from build123d import *

# Parameters (mm, degrees)
SKETCH_W             = 57
SKETCH_H             = 69
PAD_DEPTH            = 9
SKETCH001_W          = 13.25
SKETCH001_H          = 16.25
POCKET_DEPTH         = 8
SKETCH002_W          = 2
SKETCH002_H          = 51.95
SKETCH002_W_2        = 42.95
SKETCH002_H_2        = 2
POCKET015_DEPTH      = 6
BODY_PLACEMENT_ANGLE = 90


with BuildPart() as part:
    # Sketch → Pad (new body)
    with BuildSketch(Plane.XY):
        with Locations((28.5, 34.5)):
            Rectangle(SKETCH_W, SKETCH_H)
    extrude(amount=PAD_DEPTH)

    # Sketch001 (on Face6 of Pad) → Pocket (cut)
    with BuildSketch(Plane.XY.offset(9)):
        with Locations((7.425, 60.075)):
            Rectangle(SKETCH001_W, SKETCH001_H)
        with Locations((21.475, 60.075)):
            Rectangle(SKETCH001_W, SKETCH001_H)
        with Locations((35.525, 60.075)):
            Rectangle(SKETCH001_W, SKETCH001_H)
        with Locations((49.575, 60.075)):
            Rectangle(SKETCH001_W, SKETCH001_H)
        with Locations((7.425, 43.025)):
            Rectangle(SKETCH001_W, SKETCH001_H)
        with Locations((7.425, 25.975)):
            Rectangle(SKETCH001_W, SKETCH001_H)
        with Locations((7.425, 8.925)):
            Rectangle(SKETCH001_W, SKETCH001_H)
        with Locations((21.475, 43.025)):
            Rectangle(SKETCH001_W, SKETCH001_H)
        with Locations((35.525, 43.025)):
            Rectangle(SKETCH001_W, SKETCH001_H)
        with Locations((49.575, 43.025)):
            Rectangle(SKETCH001_W, SKETCH001_H)
        with Locations((21.475, 25.975)):
            Rectangle(SKETCH001_W, SKETCH001_H)
        with Locations((35.525, 25.975)):
            Rectangle(SKETCH001_W, SKETCH001_H)
        with Locations((49.575, 25.975)):
            Rectangle(SKETCH001_W, SKETCH001_H)
        with Locations((21.475, 8.925)):
            Rectangle(SKETCH001_W, SKETCH001_H)
        with Locations((35.525, 8.925)):
            Rectangle(SKETCH001_W, SKETCH001_H)
        with Locations((49.575, 8.925)):
            Rectangle(SKETCH001_W, SKETCH001_H)
    extrude(amount=-POCKET_DEPTH, mode=Mode.SUBTRACT)

    # Sketch002 (on Face5 of Pocket) → Pocket015 (cut)
    with BuildSketch(Plane.XY.offset(9)):
        with Locations((2.3, 25.975)):
            Rectangle(SKETCH002_W, SKETCH002_H)
        with Locations((16.35, 25.975)):
            Rectangle(SKETCH002_W, SKETCH002_H)
        with Locations((30.4, 25.975)):
            Rectangle(SKETCH002_W, SKETCH002_H)
        with Locations((44.45, 25.975)):
            Rectangle(SKETCH002_W, SKETCH002_H)
        with Locations((35.525, 53.45)):
            Rectangle(SKETCH002_W_2, SKETCH002_H_2)
        with Locations((35.525, 36.4)):
            Rectangle(SKETCH002_W_2, SKETCH002_H_2)
        with Locations((35.525, 19.35)):
            Rectangle(SKETCH002_W_2, SKETCH002_H_2)
        with Locations((35.525, 2.3)):
            Rectangle(SKETCH002_W_2, SKETCH002_H_2)
    extrude(amount=-POCKET015_DEPTH, mode=Mode.SUBTRACT)


with BuildPart() as part_1:
    # Body placement: moved
    add(part.part.moved(Location((75, 4, -2))).rotate(Axis((75, 4, -2), (0, 0, 1)), BODY_PLACEMENT_ANGLE))


solid = part_1.part
Verification items for the finished model (mm, model axes). A direction names the side the tool comes from. Give positions to 0.01 mm unless a question says otherwise; leave off trailing zeros. Order: outer loops, then holes, each group sorted by start corner. A loop starts at its lowest first (then second) coordinate and runs counter-clockwise, first axis right, second up. Notation, with made-up numbers: M -1.75,6 L 36.25,6 A18 ccw 36.25,28 Z; hole C 5,83 d4. An arc over 180 degrees is marked long. Use one line per item in the form item = value. Start each with the question number.
Q1. Section check A-A (y = 45). Enter the section's corners in (x, z).
Q2. Mould release check, pull along X, two halves, no side actions. Record for faces 3 (the flat face through (23.85, 41, 3)), 4 (the flat face through (27.8, 32.3, 7)), 5 (the flat face through (75, 38, 2)): +X half, -X half, draft (parallel to the pull), parting line (faces both ways), or undercut.
Q3. Scan lines: line 1 along Y through (x, z) = (13, 1); line 2 along X through (y, z) = (28, 2.75). Record each from-to range of solid material in increasing order. Write a range as [from, to].
Q4. Section check C-C (x = 15). Enter the section's corners in (y, z), then the cut area to 3 significant figures.
Q5. Go/stop test with flat-tipped pins: pin 1 Ø0.6 at (x, y) = (23.5, 34.5) entering from +Z; pin 2 Ø4 at (x, y) = (17.5, 39.5) entering from +Z. Record where each tip stops, or that it passes through.
Q6. Section check B-B (z = 2.5). Count the separate pieces of the cut face and the enclosed holes in it, then the cut area to 3 significant figures.
Q7. Access from +Z, -Z, +X, -X, +Y, -Y to the whole of each face (thin tool, end or side, straight path). Record for faces 1 (the flat face through (27.81, 18.21, 7)), 2 (the flat face through (66, 60.2, 3)).
Evaluation:
q1.outline = M 6,-2 L 75,-2 L 75,7 L 74.2,7 L 74.2,-1 L 57.95,-1 L 57.95,7 L 57.15,7 L 57.15,-1 L 40.9,-1 L 40.9,7 L 40.1,7 L 40.1,-1 L 23.85,-1 L 23.85,7 L 23.05,7 L 23.05,-1 L 6.8,-1 L 6.8,7 L 6,7 Z
q2.face_3 = undercut
q2.face_4 = draft
q2.face_5 = +X half
q3.line_1 = [4, 4.8], [18.05, 18.85], [32.1, 32.9], [46.15, 46.95], [60.2, 61]
q3.line_2 = [6, 6.8], [23.05, 23.85], [40.1, 40.9], [57.15, 57.95], [74.2, 75]
q4.outline = M 4,-2 L 61,-2 L 61,7 L 60.2,7 L 60.2,-1 L 46.95,-1 L 46.95,7 L 46.15,7 L 46.15,-1 L 32.9,-1 L 32.9,7 L 32.1,7 L 32.1,-1 L 18.85,-1 L 18.85,7 L 18.05,7 L 18.05,-1 L 4.8,-1 L 4.8,7 L 4,7 Z
q4.area = 89.0 mm2
q5.pin_1 = 1
q5.pin_2 = -1
q6.separate_pieces = 17
q6.enclosed_holes = 0
q6.area = 437 mm2
q7.face_1 = +Z, +X, -X, +Y, -Y
q7.face_2 = +Z
